```python
from build123d import *

# Parameters (mm, degrees)
F1_DEPTH = 25.4
F2_W     = 23.002351285
F2_H     = 23.5382290557
F3_DEPTH = 200
F4_W     = 22.6789787412
F4_H     = 20.0632547494
F5_DEPTH = 9.7
F6_W     = 22.6789787412
F6_H     = 20.6567810383
F7_DEPTH = 9.7


with BuildPart() as f1:
    # F0 (on Front) → F1 (new body)
    with BuildSketch(Plane.XZ):
        with BuildLine():
            Line((-88.0114324391, 44.9371878058), (-92.332277447, 44.9371878058))
            Line((-92.332277447, 44.9371878058), (-92.332277447, -3.1727263704))
            add(Edge.make_bspline(
                [(-92.332277447, -3.1727263704), (-90.1621250206, -4.8428116353), (-87.3784565002, -6.7092328778), (-81.1715490314, -8.8067426399), (-68.3223344623, -11.7452096222), (-52.7487966745, -14.6124342412), (-48.5107222082, -15.2044240054), (-42.9695285857, -15.1135046035)],
                knots=[0, 0, 0, 0, 0.1061199285, 0.2106615838, 0.3682095287, 0.5326224088, 0.6725216292, 0.6725216292, 0.6725216292, 0.6725216292], degree=3))
            Line((-42.9695285857, -15.1135046035), (-43.0925939554, -8.7688258267))
            add(Edge.make_bspline(
                [(-62.7548545599, -6.7295194604), (-59.4493670767, -7.6350430897), (-52.9059212561, -9.4275910387), (-46.3411198764, -8.9868982298), (-43.0925939554, -8.7688258267)],
                knots=[0, 0, 0, 0, 0.50516006, 1, 1, 1, 1], degree=3))
            Line((-62.7548545599, -6.7295194604), (-65.3324536979, -6.7295194604))
            add(Edge.make_bspline(
                [(-88.0114324391, 0), (-87.0734538531, -0.8836713226), (-84.3852284873, -2.9653247289), (-76.6297771142, -5.4632983452), (-68.5336425498, -5.9339730817), (-65.3324536979, -6.7295194604)],
                knots=[0, 0, 0, 0, 0.2503633507, 0.5945183664, 1, 1, 1, 1], degree=3))
            Line((-88.0114324391, 0), (-88.0114324391, 20.4308070242))
            Line((-88.0114324391, 20.4308070242), (-88.0114324391, 24.3352483958))
            Line((-88.0114324391, 24.3352483958), (-88.0114324391, 34.0071152896))
            Line((-88.0114324391, 34.0071152896), (-88.0114324391, 44.9371878058))
        make_face()
        with BuildLine():
            Line((-43.0925939554, -8.7688258267), (-42.9695285857, -15.1135046035))
            add(Edge.make_bspline(
                [(5.8930433958, -1.2674864281), (3.7892869814, -3.02047111), (1.0800895919, -4.9934354255), (-5.0408105659, -7.3300630778), (-17.7664104464, -10.764595205), (-33.2170470606, -14.233584173), (-37.4289771792, -14.989475527), (-42.9695285857, -15.1135046035)],
                knots=[0, 0, 0, 0, 0.1061199285, 0.2106615838, 0.3682095287, 0.5326224088, 0.6725216292, 0.6725216292, 0.6725216292, 0.6725216292], degree=3))
            Line((5.8930433958, -1.2674864281), (4.0274051514, 46.8062406583))
            Line((4.0274051514, 46.8062406583), (-0.2901898236, 46.6386840573))
            Line((-0.2901898236, 46.6386840573), (0.1336637968, 35.7168328718))
            Line((0.1336637968, 35.7168328718), (0.5087258829, 26.0522409176))
            Line((0.5087258829, 26.0522409176), (0.6601349068, 22.1507363704))
            Line((0.6601349068, 22.1507363704), (1.4524143278, 1.7352968948))
            add(Edge.make_bspline(
                [(1.4524143278, 1.7352968948), (0.5494088604, 0.8159166906), (-2.0560707486, -1.3684167382), (-9.7088205806, -4.1652574911), (-17.7806132945, -4.9495354876), (-20.9485440647, -5.8686213059)],
                knots=[0, 0, 0, 0, 0.2503633507, 0.5945183664, 1, 1, 1, 1], degree=3))
            Line((-20.9485440647, -5.8686213059), (-23.5242043963, -5.9685771594))
            add(Edge.make_bspline(
                [(-23.5242043963, -5.9685771594), (-26.792090576, -7.001602068), (-33.2611019617, -9.0465477999), (-39.8380549387, -8.8607607028), (-43.0925939554, -8.7688258267)],
                knots=[0, 0, 0, 0, 0.50516006, 1, 1, 1, 1], degree=3))
        make_face()
        Polygon((-24.7288546219, 25.0728245453), (-23.5242043963, -5.9685771594), (-20.9485440647, -5.8686213059), (-22.0017852664, 21.2712758516), (0.6601349068, 22.1507363704), (0.5087258829, 26.0522409176), (0.1336637968, 35.7168328718), (-22.5282563764, 34.837372353), (-22.1531942903, 25.1727803987), align=None)
        Polygon((-20.2248709389, 25.2476144923), (-20.5214146142, 32.8889456861), (-1.9144672145, 33.6110414083), (-1.6205286616, 25.9696091153), align=None, mode=Mode.SUBTRACT)
        Polygon((-65.3324536979, 34.0071152896), (-88.0114324391, 34.0071152896), (-88.0114324391, 24.3352483958), (-88.0114324391, 20.4308070242), (-65.3324536979, 20.4308070242), (-65.3324536979, -6.7295194604), (-62.7548545599, -6.7295194604), (-62.7548545599, 24.3352483958), (-65.3324536979, 24.3352483958), align=None)
        Polygon((-85.8805751163, 24.3352483958), (-85.8831821996, 31.9823315367), (-67.2622285783, 31.9823315367), (-67.2622285783, 24.3352483958), align=None, mode=Mode.SUBTRACT)
    extrude(amount=F1_DEPTH)

    # F2 (on face) → F3 (cut)
    with BuildSketch(Plane(origin=(-92.332277447, 0, 0), x_dir=(0, -1, 0), z_dir=(-1, 0, 0))):
        with Locations((12.6931375707, 8.5963881575)):
            Rectangle(F2_W, F2_H)
    extrude(amount=-F3_DEPTH, mode=Mode.SUBTRACT)

    # F4 (on face) → F5 (cut)
    with BuildSketch(Plane.XY.offset(34.0071152896)):
        with Locations((-76.6719430685, -12.7963220002)):
            Rectangle(F4_W, F4_H)
    extrude(amount=-F5_DEPTH, mode=Mode.SUBTRACT)

    # F6 (on face) → F7 (cut)
    with BuildSketch(Plane(origin=(-1.3838082935, 0, 35.6579430345), x_dir=(0.9992478247, 0, 0.038778665), z_dir=(-0.038778665, 0, 0.9992478247))):
        with Locations((-9.820875016, -12.7256970154)):
            Rectangle(F6_W, F6_H)
    extrude(amount=-F7_DEPTH, mode=Mode.SUBTRACT)


solid = f1.part
```
CAD build for the part. Positions are in the model's coordinates, mm. A direction names the side the tool comes from. Round coordinates to 2 decimals unless told otherwise and drop trailing zeros. Write item = value, one per line.
(1) Drill centre lines: L1, parallel to Z at x = -69, y = -6; L2, parallel to Z at x = -0.5, y = -18.25; L3, parallel to X at y = -18.5, z = 39. Where is each one in solid material? Low to high.
Answers follow:
L1 = -11.49 to -6.06, 20.43 to 24.31
L2 = -5.51 to -3.17, 22.11 to 25.98
L3 = -92.33 to -88.01, 0.01 to 4.33
(2) 3-axis set-ups, long thin cutter, end or side, ignore diameter. For faces 4 (the flat face through (-65.332, -1, 29)), 5 (the flat face through (-88.011, -25, 10)), 6 (the flat face through (-88.011, -13, 34)), 7 (the flat face through (-22, 0, 11)), 8 (the flat face through (2, -1.192, 8)): which of +Z, -Z, +X, -X, +Y, -Y reach the whole face in a straight line?
Answers follow:
face_4 = +Z, +Y, -Y
face_5 = +Y, -Y
face_6 = +Z
face_7 = +Z, -Z, +X, -X, +Y
face_8 = +X, -X
(3) Flat gauge pins, fed straight in: P1, Ø1, axis at x = -11.5, z = 27, coming from the +Y side; P2, Ø1.3, axis at x = 2.5, y = -17.5, coming from the -Z side; P3, Ø12, axis at x = -3.5, y = -8.5, coming from the +Z side; P4, Ø5, axis at x = -11, y = -6, coming from the -Z side. Where does each tip first touch, or does it go through?
Answers follow:
P1 = through
P2 = -4.28
P3 = 46.75
P4 = -9.57
(4) Pull direction Z, two halves, no side cores. Call faces 1 (the flat face through (-77, -13, 24.307)), 2 (the flat face through (-22, -25.4, 11)), 3 (the flat face through (-67.262, -1, 28)): +Z half, -Z half, draft (parallel to the pull), parting line (faces both ways), or undercut.
Answers follow:
face_1 = +Z half
face_2 = draft
face_3 = undercut
(5) Cut at A-A (z = 11). State how many separate pieces and enclosed holes the cut face has, plus the area to 3 significant figures.
Answers follow:
separate_pieces = 8
enclosed_holes = 0
area = 33.1 mm²
